```python
from build123d import *

# Parameters (mm, degrees)
SKETCH1_W           = 23
SKETCH1_H           = 13
BOSS_EXTRUDE1_DEPTH = 18
SKETCH2_W           = 32
SKETCH2_H           = 13
BOSS_EXTRUDE2_DEPTH = 2
SKETCH3_W           = 23
SKETCH3_H           = 13
BOSS_EXTRUDE3_DEPTH = 2
SKETCH4_W           = 15
SKETCH4_H           = 13
BOSS_EXTRUDE4_DEPTH = 6
SKETCH5_R           = 2.5
BOSS_EXTRUDE5_DEPTH = 5
SKETCH6_R           = 1
CUT_EXTRUDE1_DEPTH  = 5
SKETCH7_R           = 1
CUT_EXTRUDE2_DEPTH  = 5


with BuildPart() as part:
    # Sketch1 → Boss-Extrude1 (new body)
    with BuildSketch(Plane.XY):
        Rectangle(SKETCH1_W, SKETCH1_H)
    extrude(amount=BOSS_EXTRUDE1_DEPTH)

    # Sketch2 → Boss-Extrude2 (add)
    with BuildSketch(Plane.XY.offset(18)):
        Rectangle(SKETCH2_W, SKETCH2_H)
    extrude(amount=BOSS_EXTRUDE2_DEPTH)

    # Sketch3 → Boss-Extrude3 (add)
    with BuildSketch(Plane.XY.offset(20)):
        Rectangle(SKETCH3_W, SKETCH3_H)
    extrude(amount=BOSS_EXTRUDE3_DEPTH)

    # Sketch4 → Boss-Extrude4 (add)
    with BuildSketch(Plane.XY.offset(22)):
        with Locations((-4, 0)):
            Rectangle(SKETCH4_W, SKETCH4_H)
    extrude(amount=BOSS_EXTRUDE4_DEPTH)

    # Sketch5 → Boss-Extrude5 (add)
    with BuildSketch(Plane.XY.offset(28)):
        with Locations((-6.391509612, 0)):
            Circle(SKETCH5_R)
    extrude(amount=BOSS_EXTRUDE5_DEPTH)

    # Sketch6 → Cut-Extrude1 (cut)
    with BuildSketch(Plane.XY.offset(33)):
        with Locations((-6.391509612, 0)):
            Circle(SKETCH6_R)
    extrude(amount=-CUT_EXTRUDE1_DEPTH, mode=Mode.SUBTRACT)

    # Sketch7 → Cut-Extrude2 (cut)
    with BuildSketch(Plane.XY.offset(20)):
        with Locations((-13.689061623, 0)):
            Circle(SKETCH7_R)
        with Locations((14.201879184, 0)):
            Circle(SKETCH7_R)
    extrude(amount=-CUT_EXTRUDE2_DEPTH, mode=Mode.SUBTRACT)


solid = part.part
```
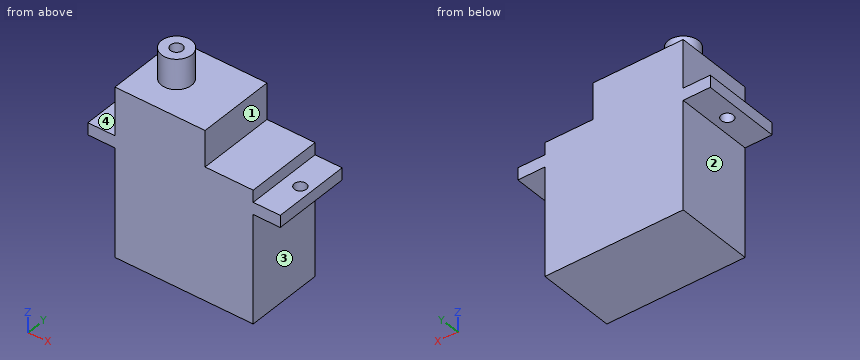
Geometry: final body of the model. Coordinates: model frame, mm. Face numbers are marked on the shaded views. A direction names the side the tool comes from. Round coordinates to 2 decimals unless told otherwise and drop trailing zeros. Write each loop counter-clockwise with the first axis right and the second up, starting at its lowest first coordinate (ties: lowest second). Pieces come first, ordered by that corner, then holes.
Item 1: Pin query (flat end, axial travel): P1, Ø5, axis at y = 2, z = 25, coming from the +X side; P2, Ø6.5, axis at y = -3, z = 11.5, coming from the +X side; P3, Ø1.5, axis at y = 3, z = 10.5, coming from the -X side. Return the tip coordinate at first contact, or that it passes through.
Item 2: Section query B-B (y = 1.75). Return loops of the section in (x, z), plus the area to 3 significant figures.
Item 3: Section query C-C (x = -11). Return loops of the section in (y, z), plus the area to 3 significant figures.
Item 4: Material intervals for L1, parallel to Z at x = 7, y = -2.75; L2, parallel to X at y = 0.5, z = 13.5; L3, parallel to Z at x = -12, y = 0.25, sorted ascending.
Item 5: Section query A-A (z = 19). Return loops of the section in (x, y).
Item 6: Section query D-D (z = 24.5). Return loops of the section in (x, y).
Item 7: Set-up query: the marked faces 1, 2, 3 and 4. Return all of +Z, -Z, +X, -X, +Y, -Y with unobstructed straight access to the full face (end or side cutting, diameter ignored); none if empty.
Completed:
1. P1: stops at x = 3.5
1. P2: stops at x = 11.5
1. P3: stops at x = -11.5
2. outline: (-16, 18) - (-11.5, 18) - (-11.5, 0) - (11.5, 0) - (11.5, 18) - (16, 18) - (16, 20) - (11.5, 20) - (11.5, 22) - (3.5, 22) - (3.5, 28) - (-4.61, 28) - (-4.61, 33) - (-8.18, 33) - (-8.18, 28) - (-11.5, 28) - (-11.5, 20) - (-16, 20) - close
2. area: 632 mm2
3. outline: (-6.5, 0) - (6.5, 0) - (6.5, 28) - (-6.5, 28) - close
3. area: 364 mm2
4. L1: z = 0 to 22
4. L2: x = -11.5 to 11.5
4. L3: z = 18 to 20
5. outline: (-16, -6.5) - (16, -6.5) - (16, 6.5) - (-16, 6.5) - close; hole circle Ø2 at (-13.69, 0); hole circle Ø2 at (14.2, 0)
6. outline: (-11.5, -6.5) - (3.5, -6.5) - (3.5, 6.5) - (-11.5, 6.5) - close
7. face 1: +Z, +X, +Y, -Y
7. face 2: -Z, -X, +Y, -Y
7. face 3: -Z, +X, +Y, -Y
7. face 4: +Z, -X, +Y, -Y
